Geometry: final body of the model. Coordinates: model frame, mm. A direction names the side the tool comes from. Give positions to 0.01 mm unless a question says otherwise; leave off trailing zeros. Order: outer loops, then holes, each group sorted by start corner. A loop starts at its lowest first (then second) coordinate and runs counter-clockwise, first axis right, second up. Notation, with made-up numbers: (51.25, -5) - (81.25, -5) arc R12 ccw to (81.25, 14) - close; hole circle Ø10 at (-4, 51). An arc over 180 degrees is marked (long way). Put each result on its own line as item: value. Start each with the question number.
1. Section B-B on x = -7. Return the cut outline in (y, z) (3 decimals), plus the area to 3 significant figures.
2. Ray query, line 1 along Y through (x, z) = (7, 7.5) (3 decimals); line 2 along X through (y, z) = (-0.5, 2.5); line 3 along Z through (x, y) = (-6.5, -0.5). Return the intervals inside material, ascending. Write a range as from..to.
3. Set-up query: faces 1 (the flat face through (0, -3.315, 5)), 2 (the flat face through (2.22, 4, 6)), 3 (the flat face through (-0.2, 4.425, 2.6)). Return all of +Z, -Z, +X, -X, +Y, -Y with unobstructed straight access to the full face (end or side cutting, diameter ignored); none if empty.
4. Section A-A on y = -2. Return the cut outline in (x, z), plus the area to 3 significant figures.
5. First-contact query: P1, Ø0.7, axis at x = 4, y = -1, coming from the +Z side. Flat tip, straight axial feed; report the tip coordinate or a pass-through.
6. Mould query, pull axis X, two halves, no side actions, for faces 4 (the flat face through (16.5, 0, 5)), 5 (the flat face through (-2.22, 4, 6)), 6 (the flat face through (0, 0, 0)). Classes: pulls with the +X half, pulls with the -X half, needs draft (parallel to the pull), parting line crosses it, or undercut.
7. Section C-C on z = 6.25. Count the separate pieces of the cut face and the enclosed holes in it, plus the area to 4 significant figures.
from build123d import *

# Parameters (mm, degrees)
SZKIC1_W                    = 33
SZKIC1_H                    = 8.85
DODANIE_WYCI_GNI_CIE1_DEPTH = 9.65
SKORUPA1_T                  = -1.11
WYTNIJ_WYCI_GNI_CIE1_REACH  = 23.064
SZKIC2_W                    = 4.44
SZKIC2_H                    = 6.81
SZKIC3_W                    = 0.6
SZKIC3_H                    = 0.6
DODANIE_WYCI_GNI_CIE2_DEPTH = 7


with BuildPart() as part:
    # Szkic1 → Dodanie-wyciągnięcie1 (new body)
    with BuildSketch(Plane.XY):
        Rectangle(SZKIC1_W, SZKIC1_H)
    extrude(amount=DODANIE_WYCI_GNI_CIE1_DEPTH)

    # Skorupa1
    skorupa1_openings = [part.faces().sort_by_distance(p)[0] for p in [
        (0, 0, 9.65),
    ]]
    offset(amount=SKORUPA1_T, openings=skorupa1_openings, kind=Kind.INTERSECTION)

    # Szkic2 → Wytnij-wyciągnięcie1 (cut, up to next)
    with BuildSketch(Plane(origin=(0, 4.425, 0), x_dir=(1, 0, 0), z_dir=(0, 1, 0)), mode=Mode.PRIVATE) as wytnij_wyci_gni_cie1_sk1:
        with Locations((0, -6.245)):
            Rectangle(SZKIC2_W, SZKIC2_H)
    wytnij_wyci_gni_cie1_tool1 = extrude(wytnij_wyci_gni_cie1_sk1.sketch, amount=-WYTNIJ_WYCI_GNI_CIE1_REACH, mode=Mode.PRIVATE) & part.part
    add(wytnij_wyci_gni_cie1_tool1.solids().sort_by_distance((0, 4.425, 6.245))[0], mode=Mode.SUBTRACT)

    # Szkic3 → Dodanie-wyciągnięcie2 (add)
    with BuildSketch(Plane.XY.offset(1.11)):
        with Locations((-11.53, 1.515)):
            Rectangle(SZKIC3_W, SZKIC3_H)
        with Locations((-8.93, 1.515)):
            Rectangle(SZKIC3_W, SZKIC3_H)
        with Locations((-6.33, 1.515)):
            Rectangle(SZKIC3_W, SZKIC3_H)
        with Locations((-3.73, 1.515)):
            Rectangle(SZKIC3_W, SZKIC3_H)
        with Locations((-1.13, 1.515)):
            Rectangle(SZKIC3_W, SZKIC3_H)
        with Locations((1.47, 1.515)):
            Rectangle(SZKIC3_W, SZKIC3_H)
        with Locations((4.07, 1.515)):
            Rectangle(SZKIC3_W, SZKIC3_H)
        with Locations((6.67, 1.515)):
            Rectangle(SZKIC3_W, SZKIC3_H)
        with Locations((9.27, 1.515)):
            Rectangle(SZKIC3_W, SZKIC3_H)
        with Locations((11.87, 1.515)):
            Rectangle(SZKIC3_W, SZKIC3_H)
        with Locations((-8.93, -1.085)):
            Rectangle(SZKIC3_W, SZKIC3_H)
        with Locations((-6.33, -1.085)):
            Rectangle(SZKIC3_W, SZKIC3_H)
        with Locations((-3.73, -1.085)):
            Rectangle(SZKIC3_W, SZKIC3_H)
        with Locations((-1.13, -1.085)):
            Rectangle(SZKIC3_W, SZKIC3_H)
        with Locations((1.47, -1.085)):
            Rectangle(SZKIC3_W, SZKIC3_H)
        with Locations((4.07, -1.085)):
            Rectangle(SZKIC3_W, SZKIC3_H)
        with Locations((6.67, -1.085)):
            Rectangle(SZKIC3_W, SZKIC3_H)
        with Locations((9.27, -1.085)):
            Rectangle(SZKIC3_W, SZKIC3_H)
        with Locations((11.87, -1.085)):
            Rectangle(SZKIC3_W, SZKIC3_H)
        with Locations((-11.53, -1.085)):
            Rectangle(SZKIC3_W, SZKIC3_H)
    extrude(amount=DODANIE_WYCI_GNI_CIE2_DEPTH)


solid = part.part
Resolved:
1. outline: (-4.425, 0) - (4.425, 0) - (4.425, 9.65) - (3.315, 9.65) - (3.315, 1.11) - (-3.315, 1.11) - (-3.315, 9.65) - (-4.425, 9.65) - close
1. area: 28.8 mm^2
2. line 1: -4.425..-3.315, 3.315..4.425
2. line 2: -16.5..-15.39, 15.39..16.5
2. line 3: 0..1.11
3. face 1: +Z
3. face 2: +Z, +Y
3. face 3: +Z, -Z, +X, -X, +Y
4. outline: (-16.5, 0) - (16.5, 0) - (16.5, 9.65) - (15.39, 9.65) - (15.39, 1.11) - (-15.39, 1.11) - (-15.39, 9.65) - (-16.5, 9.65) - close
4. area: 55.6 mm^2
5. P1: z = 8.11
6. face 4: pulls with the +X half
6. face 5: undercut
6. face 6: needs draft
7. separate pieces: 21
7. enclosed holes: 0
7. area: 90.25 mm^2
